from build123d import *

# Parameters (mm, degrees)
SKETCH1_R           = 57.15
SKETCH1_R_2         = 1.397
SKETCH1_R_3         = 3.175
BOSS_EXTRUDE1_DEPTH = 4.572
SKETCH2_R           = 2.75
SKETCH2_R_2         = 1.75
BOSS_EXTRUDE2_DEPTH = 2
SKETCH3_R           = 5
SKETCH3_R_2         = 1.75
BOSS_EXTRUDE3_DEPTH = 1.5


with BuildPart() as part:
    # Sketch1 → Boss-Extrude1 (new body)
    with BuildSketch(Plane(origin=(0, 0, 0), x_dir=(1, 0, 0), z_dir=(0, 1, 0))):
        Circle(SKETCH1_R)
        with Locations((0, 6.35)):
            Circle(SKETCH1_R_2, mode=Mode.SUBTRACT)
        with Locations((0, 25.4)):
            Circle(SKETCH1_R_3, mode=Mode.SUBTRACT)
        with Locations((0, 50.8)):
            Circle(SKETCH1_R_3, mode=Mode.SUBTRACT)
        with Locations((25.4, 0)):
            Circle(SKETCH1_R_3, mode=Mode.SUBTRACT)
        with Locations((0, -25.4)):
            Circle(SKETCH1_R_3, mode=Mode.SUBTRACT)
        with Locations((-25.4, 0)):
            Circle(SKETCH1_R_3, mode=Mode.SUBTRACT)
        with Locations((6.35, 0)):
            Circle(SKETCH1_R_2, mode=Mode.SUBTRACT)
        with Locations((0, -6.35)):
            Circle(SKETCH1_R_2, mode=Mode.SUBTRACT)
        with Locations((-6.35, 0)):
            Circle(SKETCH1_R_2, mode=Mode.SUBTRACT)
        with Locations((35.921024484, 35.921024484)):
            Circle(SKETCH1_R_3, mode=Mode.SUBTRACT)
        with Locations((50.8, 0)):
            Circle(SKETCH1_R_3, mode=Mode.SUBTRACT)
        with Locations((35.921024484, -35.921024484)):
            Circle(SKETCH1_R_3, mode=Mode.SUBTRACT)
        with Locations((0, -50.8)):
            Circle(SKETCH1_R_3, mode=Mode.SUBTRACT)
        with Locations((-35.921024484, -35.921024484)):
            Circle(SKETCH1_R_3, mode=Mode.SUBTRACT)
        with Locations((-50.8, 0)):
            Circle(SKETCH1_R_3, mode=Mode.SUBTRACT)
        with Locations((-35.921024484, 35.921024484)):
            Circle(SKETCH1_R_3, mode=Mode.SUBTRACT)
    extrude(amount=BOSS_EXTRUDE1_DEPTH)


with BuildPart() as body_2:
    # Sketch2 → Boss-Extrude2 (new body)
    with BuildSketch(Plane(origin=(0, 4.572, 0), x_dir=(1, 0, 0), z_dir=(0, 1, 0))):
        with Locations((-25.4, 0)):
            Circle(SKETCH2_R)
        with Locations((-25.4, 0)):
            Circle(SKETCH2_R_2, mode=Mode.SUBTRACT)
    extrude(amount=-BOSS_EXTRUDE2_DEPTH)

    # Sketch3 → Boss-Extrude3 (add)
    with BuildSketch(Plane(origin=(0, 4.572, 0), x_dir=(1, 0, 0), z_dir=(0, 1, 0))):
        with Locations((-25.4, 0)):
            Circle(SKETCH3_R)
        with Locations((-25.4, 0)):
            Circle(SKETCH3_R_2, mode=Mode.SUBTRACT)
    extrude(amount=BOSS_EXTRUDE3_DEPTH)


solid = body_2.part
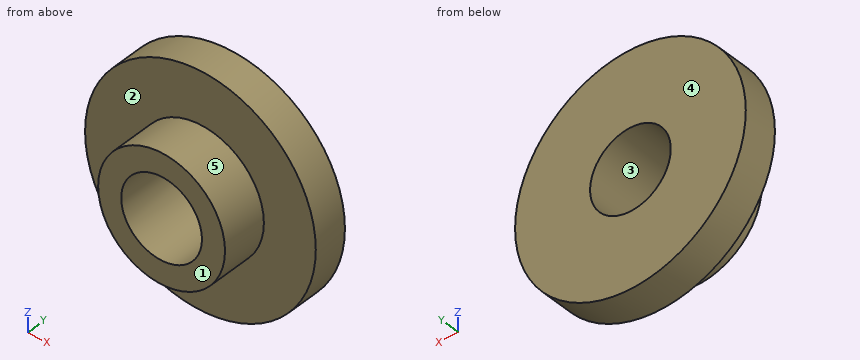
Can you work these out from the model? Positions are in its coordinate system, mm. Face numbers are marked on the shaded views. A direction names the side the tool comes from. Round coordinates to 2 decimals unless told otherwise and drop trailing zeros. Write each loop counter-clockwise with the first axis right and the second up, starting at its lowest first coordinate (ties: lowest second). Pieces come first, ordered by that corner, then holes. Notation, with made-up numbers: M -9,-23 L 26,-23 A30 ccw 26,6 Z; hole C -22,24 d11. An arc over 180 degrees is marked long. Use CSV: the item, a comma, the result in double quotes.
(1) Imagine slicing it at A-A (x = -25.4). Write out the boundary of the cut face in (y, z).
Check values:
outline,"M 2.57,-2.75 L 4.57,-2.75 L 4.57,-5 L 6.07,-5 L 6.07,-1.75 L 2.57,-1.75 Z; M 2.57,1.75 L 6.07,1.75 L 6.07,5 L 4.57,5 L 4.57,2.75 L 2.57,2.75 Z"
(2) Imagine slicing it at C-C (y = 4.2). Write out the boundary of the cut face in (x, z).
Check values:
outline,"C -25.4,0 d5.5; hole C -25.4,0 d3.5"
(3) We'd pull the mould along Z, two halves only. Please class the marked faces 3, 4 and 5: +Z half, -Z half, draft (parallel to the pull), parting line (faces both ways), or undercut.
Check values:
face 3,"undercut"
face 4,"draft"
face 5,"parting line"
(4) I need wall thicknesses on line 1 along X through (y, z) = (3.95, 0); line 2 along X through (y, z) = (4.65, 0); line 3 along Z through (x, y) = (-25.4, 4). Which ranges of each line are inside material? Lowest first, please.
Check values:
line 1,"-28.15 to -27.15, -23.65 to -22.65"
line 2,"-30.4 to -27.15, -23.65 to -20.4"
line 3,"-2.75 to -1.75, 1.75 to 2.75"
(5) I'm going to push flat-ended pins straight in: pin 1 (1 mm diameter, centred on x = -23, y = 5.5, fed in from -Z); pin 2 (5 mm diameter, centred on x = -24.5, z = 1, fed in from -Y); pin 3 (1 mm diameter, centred on x = -23, y = 3.5, fed in from +Z); pin 4 (1.5 mm diameter, centred on y = 5.5, z = -3, fed in from -X). Where does each tip first touch, or does it pass through?
Check values:
pin 1,"z = -4.62"
pin 2,"y = 2.57"
pin 3,"z = 1.99"
pin 4,"x = -29.87"
(6) Imagine slicing it at D-D (x = -28). Write out the boundary of the cut face in (y, z).
Check values:
outline,"M 2.57,-0.9 L 4.57,-0.9 L 4.57,-4.27 L 6.07,-4.27 L 6.07,4.27 L 4.57,4.27 L 4.57,0.9 L 2.57,0.9 Z"
(7) Imagine slicing it at B-B (z = 0). Write out the boundary of the cut face in (x, y).
Check values:
outline,"M -30.4,4.57 L -28.15,4.57 L -28.15,2.57 L -27.15,2.57 L -27.15,6.07 L -30.4,6.07 Z; M -23.65,2.57 L -22.65,2.57 L -22.65,4.57 L -20.4,4.57 L -20.4,6.07 L -23.65,6.07 Z"
(8) On a 3-axis mill with a long thin cutter (end or side, diameter ignored), from which of +Z, -Z, +X, -X, +Y, -Y can I reach the whole of each face in a straight line? I mean the marked faces 1 and 2. Say none if no direction works.
Check values:
face 1,"+Z, -Z, +X, -X, -Y"
face 2,"-Y"
